For this review, take the finished solid that the model builds, in its own axes (mm). A direction names the side the tool comes from. Round coordinates to 2 decimals unless told otherwise and drop trailing zeros. Loops run counter-clockwise (first coordinate to the right, second up) from the corner with the lowest first, then second, coordinate; pieces in that order, holes last.
1) Take a section at C-C (z = 22.6). State the section outline as (x, y) points.
2) Insertion check: pin 1 (3 mm diameter, centred on x = 30, y = -3.05, fed in from +Z); pin 2 (6 mm diameter, centred on x = -5.5, z = 18, fed in from +Y); pin 3 (6 mm diameter, centred on x = 11.5, y = 17.5, fed in from +Z); pin 4 (3 mm diameter, centred on x = 9, y = 0, fed in from +Z). Each pin has a flat end and moves straight along its axis. Give the tip position at first contact, or say it passes through.
3) Take a section at B-B (y = -5.5). State the section outline as (x, z) points.
4) Wall thickness on L1, parallel to Y at x = 30, z = 13.25; L2, parallel to X at y = -7.5, z = 26; L3, parallel to Z at x = 5, y = -5: over which ranges is each line inside the solid? List them lowest first.
5) Take a section at D-D (x = 30). State the section outline as (y, z) points.
6) Mouldability with a two-part tool opening along Z and no side actions: class faces 1 (the flat face through (30, 0, 20)), 2 (the cylindrical face through (-14.14, 24.1, 5.07)), 3 (the flat face through (10, 6, 0)), 4 (the flat face through (-10, 0, 23)) as pulls with the +Z half, pulls with the -Z half, needs draft (parallel to the pull), parting line crosses it, or undercut.
7) Tool access review of faces 5 (the flat face through (30, 11, 13)), 6 (the flat face through (25, 0, 15)), 7 (the cylindrical face through (-14.14, 10.1, 18.62)): name each direction out of +Z, -Z, +X, -X, +Y, -Y from which nothing blocks a thin tool from reaching the whole face with its end or side.
8) Take a section at A-A (z = 16.25). State the section outline as (x, y) points.
```python
from build123d import *

# Parameters (mm, degrees)
F0_W      = 50
F0_H      = 50
F1_DEPTH  = 10
F2_W      = 15
F2_H      = 22
F3_DEPTH  = 20
F4_R      = 4
F5_DEPTH  = 10
F6_R      = 1.65
F7_DEPTH  = 10.001
F8_W      = 10
F8_H      = 22
F9_DEPTH  = 10
F10_R     = 1.35
F11_DEPTH = 11
F12_R     = 3


with BuildPart() as f1:
    # F0 (on Top) → F1 (new body)
    with BuildSketch(Plane.XY):
        with Locations((10, 0)):
            Rectangle(F0_W, F0_H)
    extrude(amount=F1_DEPTH)

    # F2 (on face) → F3 (join)
    with BuildSketch(Plane.XY.offset(10)):
        with Locations((-7.5, 0)):
            Rectangle(F2_W, F2_H)
    extrude(amount=F3_DEPTH)

    # F4 (on face) → F5 (cut)
    with BuildSketch(Plane.YZ):
        with Locations((0, 22.6)):
            Circle(F4_R)
    extrude(amount=-F5_DEPTH, mode=Mode.SUBTRACT)

    # F6 (on face) → F7 (cut, through all)
    with BuildSketch(Plane.XY.offset(10)):
        with Locations((9, 0)):
            Circle(F6_R)
    extrude(amount=-F7_DEPTH, mode=Mode.SUBTRACT)

    # F8 (on face) → F9 (join)
    with BuildSketch(Plane.XY.offset(10)):
        with Locations((30, 0)):
            Rectangle(F8_W, F8_H)
    extrude(amount=F9_DEPTH)

    # F10 (on face) → F11 (cut)
    with BuildSketch(Plane.XY.offset(20)):
        with Locations((30, 3.05)):
            Circle(F10_R)
        with Locations((30, -3.05)):
            Circle(F10_R)
    extrude(amount=-F11_DEPTH, mode=Mode.SUBTRACT)

    # F12
    f12_edges = [f1.edges().sort_by_distance(p)[0] for p in [
        (-15, 0, 30),
        (-15, -25, 5),
        (35, -25, 5),
        (35, 25, 5),
        (-15, 25, 5),
        (-15, 11, 20),
        (-15, -11, 20),
        (-7.5, 11, 30),
        (-7.5, -11, 30),
        (30, 11, 20),
        (30, -11, 20),
    ]]
    fillet(f12_edges, radius=F12_R)


solid = f1.part
```
Response:
1. outline: (-15, -8) arc R3 ccw to (-12, -11) - (0, -11) - (0, -4) - (-10, -4) - (-10, 4) - (0, 4) - (0, 11) - (-12, 11) arc R3 ccw to (-15, 8) - close
2. pin 1: stops at z = 20
2. pin 2: stops at y = 11
2. pin 3: stops at z = 10
2. pin 4: passes through
3. outline: (-15, 0) - (35, 0) - (35, 20) - (25, 20) - (25, 10) - (0, 10) - (0, 30) - (-12, 30) arc R3 ccw to (-15, 27) - close
4. L1: y = -11 to -4.4, -1.7 to 1.7, 4.4 to 11
4. L2: x = -15 to 0
4. L3: z = 0 to 10
5. outline: (-25, 0) - (25, 0) - (25, 10) - (11, 10) - (11, 17) arc R3 ccw to (8, 20) - (4.4, 20) - (4.4, 9) - (1.7, 9) - (1.7, 20) - (-1.7, 20) - (-1.7, 9) - (-4.4, 9) - (-4.4, 20) - (-8, 20) arc R3 ccw to (-11, 17) - (-11, 10) - (-25, 10) - close
6. face 1: pulls with the +Z half
6. face 2: needs draft
6. face 3: pulls with the -Z half
6. face 4: undercut
7. face 5: +Z, +X, -X, +Y
7. face 6: +Z, +Y, -Y
7. face 7: +Z, -X, +Y
8. outline: (-15, -8) arc R3 ccw to (-12, -11) - (0, -11) - (0, 11) - (-12, 11) arc R3 ccw to (-15, 8) - close; (25, -11) - (35, -11) - (35, 11) - (25, 11) - close; hole circle Ø2.7 at (30, -3.05); hole circle Ø2.7 at (30, 3.05)
